Source: CAD feature listing. Evaluate the final solid. Frame: model axes, mm. Face numbers are marked on the shaded views. A direction names the side the tool comes from. Give positions to 0.01 mm unless a question says otherwise; leave off trailing zeros. Loops run counter-clockwise (first coordinate to the right, second up) from the corner with the lowest first, then second, coordinate; pieces in that order, holes last. Notation, with made-up numbers: M 39,-17 L 75,-17 A7 cw 75,-7 Z; hole C -27.5,16 d11. An arc over 180 degrees is marked long. Answer in a Markdown table with one row per item.
```python
from build123d import *

# Parameters (mm, degrees)
F0_R     = 25.4
F0_R_2   = 3.556
F1_DEPTH = 6.35
F3_DEPTH = 76.2


with BuildPart() as f1:
    # F0 (on Right) → F1 (new body)
    with BuildSketch(Plane.YZ):
        Circle(F0_R)
        Circle(F0_R_2, mode=Mode.SUBTRACT)
    extrude(amount=F1_DEPTH)

    # F2 (on face) → F3 (cut)
    with BuildSketch(Plane(origin=(0, 0, 0), x_dir=(0, -1, 0), z_dir=(-1, 0, 0))):
        with BuildLine():
            Line((-3.376935, 12.234649), (-2.113646, 7.640875))
            Line((-2.113646, 7.640875), (1.905905, 7.640875))
            Line((1.905905, 7.640875), (3.398881, 12.579182))
            ThreePointArc((3.398881, 12.579182), (-0.096865, 14.52771), (-3.376935, 12.234649))
        make_face()
    extrude(amount=-F3_DEPTH, mode=Mode.SUBTRACT)


solid = f1.part
```
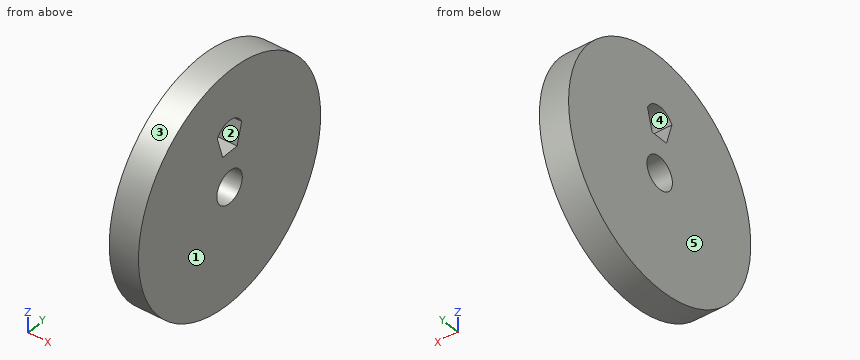
1) Pull-direction query (Y, two-part tool) for the marked faces 3, 4 and 5; classes: released by +Y, released by -Y, zero draft, split by the parting line, or undercut.
Reply:
| item | result |
|---|---|
| face 3 | split by the parting line |
| face 4 | undercut |
| face 5 | zero draft |
2) Section D-D, the plane z = -14.5. Return loops of the section in (x, y).
Reply:
| item | result |
|---|---|
| outline | M 0,-20.85 L 6.35,-20.85 L 6.35,20.85 L 0,20.85 Z |
3) Set-up query: the marked faces 1 and 2. Return all of +Z, -Z, +X, -X, +Y, -Y with unobstructed straight access to the full face (end or side cutting, diameter ignored); none if empty.
Reply:
| item | result |
|---|---|
| face 1 | +Z, -Z, +X, +Y, -Y |
| face 2 | +X, -X |
4) Pin query (flat end, axial travel): pin 1 Ø2 at (x, y) = (3, 0.5) entering from +Z; pin 2 Ø2 at (x, y) = (2.5, -3.5) entering from +Z. Return the tip coordinate at first contact, or that it passes through.
Reply:
| item | result |
|---|---|
| pin 1 | stops at z = 25.4 |
| pin 2 | stops at z = 25.28 |
5) Section A-A, the plane z = 0. Return loops of the section in (x, y).
Reply:
| item | result |
|---|---|
| outline | M 0,-25.4 L 6.35,-25.4 L 6.35,-3.56 L 0,-3.56 Z; M 0,3.56 L 6.35,3.56 L 6.35,25.4 L 0,25.4 Z |
6) Material intervals for L1, parallel to Z at x = 3, y = 0; L2, parallel to Z at x = 2, y = -0.5; L3, parallel to Y at x = 1, z = -3, sorted ascending.
Reply:
| item | result |
|---|---|
| L1 | z = -25.4 to -3.56, 3.56 to 7.64, 14.53 to 25.4 |
| L2 | z = -25.4 to -3.52, 3.52 to 7.64, 14.51 to 25.4 |
| L3 | y = -25.22 to -1.91, 1.91 to 25.22 |
7) Section B-B, the plane x = 4.25. Return loops of the section in (y, z), then the cut area to 3 significant figures.
Reply:
| item | result |
|---|---|
| outline | C 0,0 d50.8; hole C 0,0 d7.11; hole M -3.4,12.58 L -1.91,7.64 L 2.11,7.64 L 3.38,12.23 A3.77 ccw Z |
| area | 1,950 mm² |
8) Section C-C, the plane y = 0. Return loops of the section in (x, z).
Reply:
| item | result |
|---|---|
| outline | M 0,-25.4 L 6.35,-25.4 L 6.35,-3.56 L 0,-3.56 Z; M 0,3.56 L 6.35,3.56 L 6.35,7.64 L 0,7.64 Z; M 0,14.53 L 6.35,14.53 L 6.35,25.4 L 0,25.4 Z |
